The listing builds one solid part. Answer for the finished solid, in the listing's coordinates (mm). Face numbers are marked on the shaded views. A direction names the side the tool comes from. Round coordinates to 2 decimals unless told otherwise and drop trailing zeros. Loops run counter-clockwise (first coordinate to the right, second up) from the corner with the lowest first, then second, coordinate; pieces in that order, holes last. Notation, with made-up numbers: (-8, 6.5) -> (50, 6.5) arc R24 cw to (50, 26.5) -> close; hole circle Ø8 at (-8.75, -16.75). An arc over 180 degrees is marked (long way). Answer in a Markdown table with one row per item. Add a question column.
```python
from build123d import *

# Parameters (mm, degrees)
SKETCH1_W           = 43.5
SKETCH1_H           = 18
BOSS_EXTRUDE1_DEPTH = 2
SKETCH2_W           = 7.549869754
SKETCH2_H           = 7.6
BOSS_EXTRUDE2_DEPTH = 4
BOSS_EXTRUDE3_DEPTH = 1
CUT_EXTRUDE1_DEPTH  = 15
CUT_EXTRUDE2_DEPTH  = 8


with BuildPart() as part:
    # Sketch1 → Boss-Extrude1 (new body)
    with BuildSketch(Plane(origin=(0, 0, 0), x_dir=(1, 0, 0), z_dir=(0, 1, 0))):
        Rectangle(SKETCH1_W, SKETCH1_H)
    extrude(amount=BOSS_EXTRUDE1_DEPTH)

    # Sketch2 → Boss-Extrude2 (add)
    with BuildSketch(Plane(origin=(0, 2, 0), x_dir=(1, 0, 0), z_dir=(0, 1, 0))):
        with Locations((-17.975065123, 0)):
            Rectangle(SKETCH2_W, SKETCH2_H)
    extrude(amount=BOSS_EXTRUDE2_DEPTH)

    # Sketch3 → Boss-Extrude3 (add)
    with BuildSketch(Plane.ZY.offset(21.75)):
        with BuildLine():
            ThreePointArc((-3.8, 3.623606798), (-3.770130162, 3.518460575), (-3.689442719, 3.44472136))
            Line((-3.689442719, 3.44472136), (-2.910557281, 3.05527864))
            ThreePointArc((-2.910557281, 3.05527864), (-2.829869838, 2.981539425), (-2.8, 2.876393202))
            Line((-2.8, 2.876393202), (-2.8, 2.2))
            ThreePointArc((-2.8, 2.2), (-2.741421356, 2.058578644), (-2.6, 2))
            Line((-2.6, 2), (2.6, 2))
            ThreePointArc((2.6, 2), (2.741421356, 2.058578644), (2.8, 2.2))
            Line((2.8, 2.2), (2.8, 2.876393202))
            ThreePointArc((2.8, 2.876393202), (2.829869838, 2.981539425), (2.910557281, 3.05527864))
            Line((2.910557281, 3.05527864), (3.689442719, 3.44472136))
            ThreePointArc((3.689442719, 3.44472136), (3.770130162, 3.518460575), (3.8, 3.623606798))
            Line((3.8, 3.623606798), (3.8, 5.8))
            ThreePointArc((3.8, 5.8), (3.741421356, 5.941421356), (3.6, 6))
            Line((3.6, 6), (-3.6, 6))
            ThreePointArc((-3.6, 6), (-3.741421356, 5.941421356), (-3.8, 5.8))
            Line((-3.8, 5.8), (-3.8, 3.623606798))
        make_face()
    extrude(amount=BOSS_EXTRUDE3_DEPTH)

    # Sketch6 → Cut-Extrude1 (cut)
    with BuildSketch(Plane.ZY.offset(22.75)):
        with BuildLine():
            Line((-2.910557281, 3.05527864), (-3.689442719, 3.44472136))
            ThreePointArc((-3.689442719, 3.44472136), (-3.770130162, 3.518460575), (-3.8, 3.623606798))
            Line((-3.8, 3.623606798), (-3.8, 2))
            Line((-3.8, 2), (-2.6, 2))
            ThreePointArc((-2.6, 2), (-2.741421356, 2.058578644), (-2.8, 2.2))
            Line((-2.8, 2.2), (-2.8, 2.876393202))
            ThreePointArc((-2.8, 2.876393202), (-3.170130162, 2.77124698), (-2.910557281, 3.05527864))
        make_face()
        with BuildLine():
            Line((-3.8, 6), (-3.8, 5.8))
            ThreePointArc((-3.8, 5.8), (-3.741421356, 5.941421356), (-3.6, 6))
            Line((-3.6, 6), (-3.8, 6))
        make_face()
        with BuildLine():
            ThreePointArc((-2.8, 2.876393202), (-2.829869838, 2.981539425), (-2.910557281, 3.05527864))
            ThreePointArc((-2.910557281, 3.05527864), (-3.170130162, 2.77124698), (-2.8, 2.876393202))
        make_face()
        with BuildLine():
            ThreePointArc((2.910557281, 3.05527864), (2.829869838, 2.981539425), (2.8, 2.876393202))
            ThreePointArc((2.8, 2.876393202), (3, 2.676393202), (3.2, 2.876393202))
            ThreePointArc((3.2, 2.876393202), (3.105146222, 3.046523364), (2.910557281, 3.05527864))
        make_face()
        with BuildLine():
            ThreePointArc((2.8, 2.2), (2.741421356, 2.058578644), (2.6, 2))
            Line((2.6, 2), (3.8, 2))
            Line((3.8, 2), (3.8, 3.623606798))
            ThreePointArc((3.8, 3.623606798), (3.770130162, 3.518460575), (3.689442719, 3.44472136))
            Line((3.689442719, 3.44472136), (2.910557281, 3.05527864))
            ThreePointArc((2.910557281, 3.05527864), (3.105146222, 3.046523364), (3.2, 2.876393202))
            ThreePointArc((3.2, 2.876393202), (3, 2.676393202), (2.8, 2.876393202))
            Line((2.8, 2.876393202), (2.8, 2.2))
        make_face()
        with BuildLine():
            Line((3.8, 6), (3.6, 6))
            ThreePointArc((3.6, 6), (3.741421356, 5.941421356), (3.8, 5.8))
            Line((3.8, 5.8), (3.8, 6))
        make_face()
    extrude(amount=-CUT_EXTRUDE1_DEPTH, mode=Mode.SUBTRACT)

    # Sketch7 → Cut-Extrude2 (cut)
    with BuildSketch(Plane.ZY.offset(22.75)):
        with BuildLine():
            Line((3.1, 5.3), (-3.1, 5.3))
            Line((-3.1, 5.3), (-3.1, 3.932623792))
            Line((-3.1, 3.932623792), (-2.597507764, 3.681377674))
            ThreePointArc((-2.597507764, 3.681377674), (-2.234414272, 3.349551203), (-2.1, 2.876393202))
            Line((-2.1, 2.876393202), (-2.1, 2.7))
            Line((-2.1, 2.7), (2.1, 2.7))
            Line((2.1, 2.7), (2.1, 2.876393202))
            ThreePointArc((2.1, 2.876393202), (2.234414272, 3.349551203), (2.597507764, 3.681377674))
            Line((2.597507764, 3.681377674), (3.1, 3.932623792))
            Line((3.1, 3.932623792), (3.1, 5.3))
        make_face()
    extrude(amount=-CUT_EXTRUDE2_DEPTH, mode=Mode.SUBTRACT)


solid = part.part
```
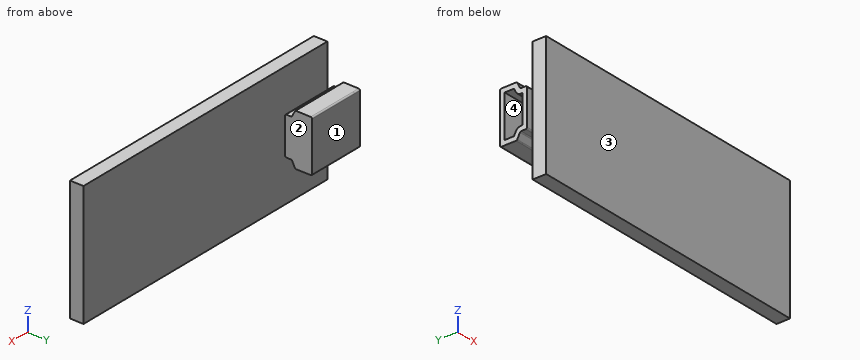
Item 1: For the marked faces 1 and 2, determine the directions among +Z, -Z, +X, -X, +Y, -Y from which every point of the face is accessible in a straight line to the end or side of a thin tool.
Item 2: Flat-ended cylindrical pins translate along their axes: P1, Ø10, axis at x = 1.5, z = -6, coming from the +Y side; P2, Ø1.3, axis at y = 4, z = 0.5, coming from the -X side; P3, Ø1.6, axis at y = 1, z = -1.5, coming from the -X side. Find the tip coordinate at first contact, or state that the pin passes through.
Item 3: Consider L1, parallel to Y at x = -15, z = 2; L2, parallel to X at y = 3.6, z = 2.75; L3, parallel to Y at x = 13, z = -1.5. Determine where each line is inside the solid, lowest interval first. Write a range as from..to.
Item 4: Section B-B, the plane z = -1.25 is taken. Write down the section's boundary in (x, y), and give its area (3 significant figures).
Item 5: Section D-D, the plane x = 4 is taken. Write down the section's boundary in (y, z), and give its area (3 significant figures).
Item 6: Section C-C, the plane y = 1.05 is taken. Write down the section's boundary in (x, z), and give its area (3 significant figures).
Item 7: The mould has two halves that part along Z. Classify the marked faces 3 and 4: +Z half, -Z half, draft (parallel to the pull), parting line (faces both ways), or undercut.
Here are the results:
| question | item | result |
|---|---|---|
| 1 | face 1 | +Z, -Z, +X, -X, +Y |
| 1 | face 2 | +Z, -Z, +X, +Y |
| 2 | P1 | stops at y = 2 |
| 2 | P2 | stops at x = -14.75 |
| 2 | P3 | stops at x = -21.75 |
| 3 | L1 | y = 0..2.7, 5.3..6 |
| 3 | L2 | x = -22.75..-14.2 |
| 3 | L3 | y = 0..2 |
| 4 | outline | (-22.75, 2) -> (-21.75, 2) -> (-21.75, 0) -> (21.75, 0) -> (21.75, 2) -> (-14.2, 2) -> (-14.2, 6) -> (-22.75, 6) -> (-22.75, 5.3) -> (-14.75, 5.3) -> (-14.75, 2.7) -> (-22.75, 2.7) -> close |
| 4 | area | 100 mm² |
| 5 | outline | (0, -9) -> (2, -9) -> (2, 9) -> (0, 9) -> close |
| 5 | area | 36.0 mm² |
| 6 | outline | (-21.75, -9) -> (21.75, -9) -> (21.75, 9) -> (-21.75, 9) -> close |
| 6 | area | 783 mm² |
| 7 | face 3 | draft |
| 7 | face 4 | undercut |
